```python
from build123d import *

# Parameters (mm, degrees)
SKETCH009_R                       = 3.25
EXTRUDE003_DEPTH                  = 3
SKETCH008_R                       = 3.25
EXTRUDE002_DEPTH                  = 10
SKETCH007_R                       = 1.75
SKETCH007_R_2                     = 1.3
EXTRUDE001_DEPTH                  = 25
EXTRUDE_DEPTH                     = 46
EXTRUDE_ONTO_SKETCH003_ROLL_ANGLE = 90
CHAMFER_SIZE                      = 0.7


with BuildPart() as extrude003:
    # Sketch009 → Extrude003 (new body)
    with BuildSketch(Plane.XY):
        with Locations((0, 20)):
            Circle(SKETCH009_R)
    extrude(amount=EXTRUDE003_DEPTH)


with BuildPart() as extrude002:
    # Sketch008 → Extrude002 (new body)
    with BuildSketch(Plane.XY):
        with Locations((-16, 5)):
            Circle(SKETCH008_R)
        with Locations((16, 5)):
            Circle(SKETCH008_R)
        with Locations((-16, 35)):
            Circle(SKETCH008_R)
        with Locations((16, 35)):
            Circle(SKETCH008_R)
    extrude(amount=EXTRUDE002_DEPTH)


with BuildPart() as extrude001:
    # Sketch007 → Extrude001 (new body)
    with BuildSketch(Plane.XY):
        with Locations((-16, 5)):
            Circle(SKETCH007_R)
        with Locations((16, 5)):
            Circle(SKETCH007_R)
        with Locations((-16, 35)):
            Circle(SKETCH007_R)
        with Locations((16, 35)):
            Circle(SKETCH007_R)
        with Locations((0, 20)):
            Circle(SKETCH007_R_2)
    extrude(amount=EXTRUDE001_DEPTH)


with BuildPart() as chamfer_body:
    # Sketch003 as drawn → Extrude (new)
    with BuildSketch(Plane.XY):
        with BuildLine():
            Line((21, 16.128044), (21, 7))
            Line((14, 7), (21, 7))
            Line((5.5, 0), (14, 7))
            Line((-5.5, 0), (5.5, 0))
            Line((-5.5, 0), (-14, 7))
            Line((-14, 7), (-21, 7))
            Line((-21, 7), (-21, 17))
            Line((-21, 17), (-12.5, 17))
            ThreePointArc((-12.5, 17), (-0.436244, 4.507615), (12.469551, 16.128044))
            Line((12.469551, 16.128044), (21, 16.128044))
        make_face()
    extrude(amount=-EXTRUDE_DEPTH)


with BuildPart() as chamfer_body_1:
    # Extrude onto Sketch003 roll: moved
    add(chamfer_body.part.rotate(Axis((0, 0, 0), (1, 0, 0)), EXTRUDE_ONTO_SKETCH003_ROLL_ANGLE))


with BuildPart() as chamfer_body_2:
    # Extrude onto Sketch003 placement: moved
    add(chamfer_body_1.part)

    # Cut: cut Extrude001
    add(extrude001.part, mode=Mode.SUBTRACT)

    # Cut001: cut Extrude002
    add(extrude002.part, mode=Mode.SUBTRACT)

    # Cut002: cut Extrude003
    add(extrude003.part, mode=Mode.SUBTRACT)

    # Chamfer
    chamfer_edges = [chamfer_body_2.edges().sort_by_distance(p)[0] for p in [
        (-16.75, 0, 17),
        (-0.436244, 0, 4.507615),
        (16.734775, 0, 16.128044),
        (-16.75, 46, 17),
        (-0.436244, 46, 4.507615),
        (16.734775, 46, 16.128044),
        (-21, 23, 17),
        (-12.5, 23, 17),
        (12.469551, 23, 16.128044),
        (21, 23, 16.128044),
    ]]
    chamfer(chamfer_edges, length=CHAMFER_SIZE)


solid = chamfer_body_2.part
```
CAD build for the part. Positions are in the model's coordinates, mm. A direction names the side the tool comes from. Round coordinates to 2 decimals unless told otherwise and drop trailing zeros. Loops run counter-clockwise (first coordinate to the right, second up) from the corner with the lowest first, then second, coordinate; pieces in that order, holes last. Notation, with made-up numbers: M 37.5,36 L 96.5,36 A16 cw 96.5,62 Z; hole C 69,18.5 d3. An arc over 180 degrees is marked long. Use a Markdown table: item, result. Add a question column.
(1) Drill centre lines: line 1 (Y direction, x = -16, z = 14); line 2 (Y direction, x = 16, z = 7.85); line 3 (X direction, y = 36.5, z = 10.5). Where is each one in solid material? Low to high.
(2) Pull direction X, two halves, no side cores. Call faces 5 (the face through (9.69, 22.68, 3.45)), 6 (the face through (-0.68, 45.41, 4.41)), 7 (the face through (0, 46, 3)), 8 (the face through (-9.69, 22.68, 3.45)): +X half, -X half, draft (parallel to the pull), parting line (faces both ways), or undercut.
(3) Cut at C-C (y = 35). Give the cut face in (x, z), and give its area (3 significant figures).
(4) Flat gauge pins, fed straight in: pin 1 (3.5 mm diameter, centred on x = 17, y = 22, fed in from +Z); pin 2 (5.5 mm diameter, centred on x = -16, y = 5, fed in from -Z); pin 3 (4 mm diameter, centred on x = -5.5, y = 37, fed in from +Z); pin 4 (5 mm diameter, centred on x = 1, y = 19, fed in from -Z). Where does each tip first touch, or does it go through?
(5) Cut at A-A (x = 0). Give the cut face in (y, z).
(6) Which spindle directions (+Z, -Z, +X, -X, +Y, -Y) get a long thin tool onto all of the face, cutting with end or side? Do faces 1 (the face through (-18, 23, 7)), 2 (the face through (-17, 23, 17)), 3 (the face through (18, 23, 7)), 4 (the face through (-12.9, 35.98, 8.4)). Say none if no direction does.
(7) Cut at B-B (y = 20). Give the cut face in (x, z), and give its area (3 significant figures).
(8) Cut at D-D (z = 14.5). State how many separate pieces and enclosed holes the cut face has, and give its area (3 significant figures).
Geometry says:
| question | item | result |
|---|---|---|
| 1 | line 1 | y = 0 to 3.25, 6.75 to 33.25, 36.75 to 46 |
| 1 | line 2 | y = 0 to 1.75, 8.25 to 31.75, 38.25 to 46 |
| 1 | line 3 | x = -21 to -16.9, -15.1 to -10.68, 10.68 to 15.1, 16.9 to 21 |
| 2 | face 5 | +X half |
| 2 | face 6 | undercut |
| 2 | face 7 | draft |
| 2 | face 8 | -X half |
| 3 | outline | M -21,7 L -19.25,7 L -19.25,10 L -17.75,10 L -17.75,17 L -20.3,17 L -21,16.3 Z; M -14.25,10 L -12.75,10 L -12.75,5.97 L -5.5,0 L 5.5,0 L 12.75,5.97 L 12.75,10 L 14.25,10 L 14.25,16.13 L 13.17,16.13 L 12.4,15.43 A12.5 cw -12.48,16.3 L -13.2,17 L -14.25,17 Z; M 17.75,10 L 19.25,10 L 19.25,7 L 21,7 L 21,15.43 L 20.3,16.13 L 17.75,16.13 Z |
| 3 | area | 216 mm² |
| 4 | pin 1 | stops at z = 16.13 |
| 4 | pin 2 | stops at z = 10 |
| 4 | pin 3 | stops at z = 7 |
| 4 | pin 4 | stops at z = 0 |
| 5 | outline | M 0,0 L 16.75,0 L 16.75,3 L 18.7,3 L 18.7,4.5 L 0.7,4.5 L 0,3.8 Z; M 21.3,3 L 23.25,3 L 23.25,0 L 46,0 L 46,3.8 L 45.3,4.5 L 21.3,4.5 Z |
| 6 | face 1 | -Z, -X, +Y, -Y |
| 6 | face 2 | +Z, +X, -X, +Y, -Y |
| 6 | face 3 | -Z, +X, +Y, -Y |
| 6 | face 4 | -Z |
| 7 | outline | M -21,7 L -14,7 L -5.5,0 L -3.25,0 L -3.25,3 L -1.3,3 L -1.3,4.57 A12.5 cw -12.48,16.3 L -13.2,17 L -20.3,17 L -21,16.3 Z; M 1.3,3 L 3.25,3 L 3.25,0 L 5.5,0 L 14,7 L 21,7 L 21,15.43 L 20.3,16.13 L 13.17,16.13 L 12.4,15.43 A12.5 cw 1.3,4.57 Z |
| 7 | area | 279 mm² |
| 8 | separate pieces | 2 |
| 8 | enclosed holes | 4 |
| 8 | area | 766 mm² |
